from build123d import *

# Parameters (mm, degrees)
SKETCH1_W           = 12.7
SKETCH1_H           = 25.4
BOSS_EXTRUDE1_DEPTH = 2.54
CUT_EXTRUDE1_REACH  = 16.424
SKETCH2_R           = 1.524
SKETCH2_R_2         = 1.26365


with BuildPart() as part:
    # Sketch1 → Boss-Extrude1 (new body)
    with BuildSketch(Plane.XY):
        Rectangle(SKETCH1_W, SKETCH1_H)
    extrude(amount=BOSS_EXTRUDE1_DEPTH)

    # Sketch2 → Cut-Extrude1 (cut, up to next)
    with BuildSketch(Plane.XY.offset(2.54), mode=Mode.PRIVATE) as cut_extrude1_sk1:
        with Locations((3.55, 7.501932673)):
            Circle(SKETCH2_R)
    cut_extrude1_tool1 = extrude(cut_extrude1_sk1.sketch, amount=-CUT_EXTRUDE1_REACH, mode=Mode.PRIVATE) & part.part
    # Sketch2 → Cut-Extrude1 (cut, up to next)
    with BuildSketch(Plane.XY.offset(2.54), mode=Mode.PRIVATE) as cut_extrude1_sk2:
        with Locations((3.55, -5.498067327)):
            Circle(SKETCH2_R_2)
    cut_extrude1_tool2 = extrude(cut_extrude1_sk2.sketch, amount=-CUT_EXTRUDE1_REACH, mode=Mode.PRIVATE) & part.part
    add(cut_extrude1_tool1.solids().sort_by_distance((3.55, 7.501933, 2.54))[0], mode=Mode.SUBTRACT)
    add(cut_extrude1_tool2.solids().sort_by_distance((3.55, -5.498067, 2.54))[0], mode=Mode.SUBTRACT)


solid = part.part
Can you work these out from the model? Positions are in its coordinate system, mm. Give positions to 0.01 mm unless a question says otherwise; leave off trailing zeros. Order: outer loops, then holes, each group sorted by start corner. A loop starts at its lowest first (then second) coordinate and runs counter-clockwise, first axis right, second up. Notation, with made-up numbers: (45, 79) - (84, 79) arc R22 cw to (84, 103) - close; hole circle Ø2 at (81.5, 49). An arc over 180 degrees is marked (long way). Write each question's results on one line, items separated by ' | '.
1) Suppose I cut it at B-B, the plane y = 8.5. Write out the boundary of the cut face in (x, z).
Final values:
outline: (-6.35, 0) - (2.4, 0) - (2.4, 2.54) - (-6.35, 2.54) - close; (4.7, 0) - (6.35, 0) - (6.35, 2.54) - (4.7, 2.54) - close
2) Suppose I cut it at C-C, the plane z = 1.75. Write out the boundary of the cut face in (x, y), then the cut area to 3 significant figures.
Final values:
outline: (-6.35, -12.7) - (6.35, -12.7) - (6.35, 12.7) - (-6.35, 12.7) - close; hole circle Ø3.05 at (3.55, 7.5); hole circle Ø2.53 at (3.55, -5.5) | area: 310 mm^2
3) Please list where these lines run through material, in increasing order: line 1 along Y through (x, z) = (3.55, 1.7); line 2 along Y through (x, z) = (3.75, 0.55); line 3 along X through (y, z) = (-6.5, 2.3). Write a range as [from, to].
Final values:
line 1: y = [-12.7, -6.76], [-4.23, 5.98], [9.03, 12.7] | line 2: y = [-12.7, -6.75], [-4.25, 5.99], [9.01, 12.7] | line 3: x = [-6.35, 2.78], [4.32, 6.35]
4) If we mould it in two halves opening along Y, with no side actions, what happens to faces 1 (the face through (0, 12.7, 1)), 2 (the face through (2.4, 8.5, 1.3)), 3 (the face through (0, 0, 2.54))? For each: pulls with the +Y half, pulls with the -Y half, needs draft (parallel to the pull), parting line crosses it, or undercut.
Final values:
face 1: pulls with the +Y half | face 2: undercut | face 3: needs draft
5) I'm going to push a flat-ended pin straight in: pin 1 Ø1.5 at (x, y) = (3.55, -5.5) entering from -Z. Where does the tip first touch, or does it pass through?
Final values:
pin 1: passes through
6) Suppose I cut it at A-A, the plane x = 3.55. Write out the boundary of the cut face in (y, z), then the cut area to 3 significant figures.
Final values:
outline: (-12.7, 0) - (-6.76, 0) - (-6.76, 2.54) - (-12.7, 2.54) - close; (-4.23, 0) - (5.98, 0) - (5.98, 2.54) - (-4.23, 2.54) - close; (9.03, 0) - (12.7, 0) - (12.7, 2.54) - (9.03, 2.54) - close | area: 50.4 mm^2
